from build123d import *

# Parameters (mm, degrees)
BOSS_EXTRUDE1_START = -1.5748
BOSS_EXTRUDE1_DEPTH = 126.1872
SKETCH2_R           = 5.499987026
CUT_EXTRUDE1_DEPTH  = 63.5


with BuildPart() as part:
    # Sketch1 → Boss-Extrude1 (new body)
    with BuildSketch(Plane.XY.offset(BOSS_EXTRUDE1_START)):
        with BuildLine():
            Line((5.5372, 43.3324), (35.215013396, -3.286034747))
            ThreePointArc((35.215013396, -3.286034747), (36.732607503, -7.536738968), (36.259288034, -12.025340858))
            Line((36.259288034, -12.025340858), (35.882961927, -13.127438743))
            ThreePointArc((35.882961927, -13.127438743), (33.545277751, -16.934256169), (29.80068515, -19.370370386))
            Line((29.80068515, -19.370370386), (5.435919899, -28.405771229))
            Line((5.435919899, -28.405771229), (5.401855854, -25.709375395))
            Line((5.401855854, -25.709375395), (28.91752571, -16.988852088))
            ThreePointArc((28.91752571, -16.988852088), (31.725970161, -15.161766425), (33.479233293, -12.306653356))
            Line((33.479233293, -12.306653356), (33.8555594, -11.204555471))
            ThreePointArc((33.8555594, -11.204555471), (34.210549002, -7.838104053), (33.072353421, -4.650075887))
            Line((33.072353421, -4.650075887), (3.394540025, 41.96835886))
            Line((3.394540025, 41.96835886), (5.5372, 43.3324))
        make_face()
    extrude(amount=-BOSS_EXTRUDE1_DEPTH)

    # Sketch2 → Cut-Extrude1 (cut)
    with BuildSketch(Plane(origin=(23.570559322, 15.005279885, 0), x_dir=(0, 0, -1), z_dir=(0.843566919, 0.537024071, 0))):
        with Locations((64.6684, 15.22665607)):
            Circle(SKETCH2_R)
    extrude(amount=-CUT_EXTRUDE1_DEPTH, mode=Mode.SUBTRACT)


solid = part.part
Read the model definition and answer for the solid it produces. Units are mm, in the model's axes. A direction names the side the tool comes from. Coordinates: 2 decimals unless noted, no trailing zeros. Write each loop counter-clockwise with the first axis right and the second up, starting at its lowest first coordinate (ties: lowest second). Pieces come first, ordered by that corner, then holes. Notation, with made-up numbers: M -38.75,-27 L -4.75,-27 A22 ccw -4.75,-6 Z; hole C 25.25,19 d11. An arc over 180 degrees is marked long. Use a Markdown table: item, result.
Q1. The part is cut by section C-C, the plane y = -22. Write down the section's boundary in (x, z), then the cut area to 3 significant figures.
Answer block:
| item | result |
|---|---|
| outline | M 15.4,-127.76 L 22.71,-127.76 L 22.71,-1.57 L 15.4,-1.57 Z |
| area | 922 mm2 |
Q2. Each of these flat-tipped pins is pushed along its axis until it touches: pin 1 Ø8 at (y, z) = (-8.5, -77.5) entering from -X; pin 2 Ø10 at (x, z) = (15, -48) entering from -Y; pin 3 Ø1 at (x, z) = (27.5, -64.5) entering from -Y. Where does it stop, or does it pass through?
Answer block:
| item | result |
|---|---|
| pin 1 | stops at x = 32.98 |
| pin 2 | stops at y = -26.71 |
| pin 3 | stops at y = -20.41 |
Q3. The part is cut by section B-B, the plane z = -73. Write down the section's boundary in (x, y), then the cut area to 3 significant figures.
Answer block:
| item | result |
|---|---|
| outline | M 3.39,41.97 L 33.07,-4.65 A7.62 cw 33.86,-11.2 L 33.48,-12.31 A7.62 cw 28.92,-16.99 L 5.4,-25.71 L 5.44,-28.41 L 29.8,-19.37 A10.16 ccw 35.88,-13.13 L 36.26,-12.03 A10.16 ccw 35.22,-3.29 L 5.54,43.33 Z |
| area | 248 mm2 |
Q4. Straight lines are drawn through the part: L1, parallel to Y at x = 27.5, z = -121.5; L2, parallel to Y at x = 21, z = -42.5; L3, parallel to X at y = -4.5, z = -35.5. For each, find the intervals that lie inside material, in ascending order. Write a range as [from, to].
Answer block:
| item | result |
|---|---|
| L1 | y = [-20.22, -17.51], [4.1, 8.83] |
| L2 | y = [-22.63, -19.92], [14.31, 19.04] |
| L3 | x = [32.98, 35.88] |
Q5. Determine the mould class of faces 1 (the face through (28, 5, -1.575)), 2 (the face through (36.725, -7.473, -63.785)), 3 (the face through (13.4, 28.6, -69.9)) for opening direction Z: released by +Z, released by -Z, zero draft, split by the parting line, or undercut.
Answer block:
| item | result |
|---|---|
| face 1 | released by +Z |
| face 2 | zero draft |
| face 3 | undercut |
Q6. Which of the six approach directions +Z, -Z, +X, -X, +Y, -Y give full straight-line access (tool end or side, diameter ignored) to faces 4 (the face through (17, -21.41, -63.79)), 5 (the face through (28, 5, -127.762))?
Answer block:
| item | result |
|---|---|
| face 4 | +Z, -Z, -X |
| face 5 | -Z, +X, -X, +Y, -Y |
Q7. The part is cut by section D-D, the plane y = 0. Write down the section's boundary in (x, z).
Answer block:
| item | result |
|---|---|
| outline | M 30.11,-127.76 L 33.12,-127.76 L 33.12,-1.57 L 30.11,-1.57 Z |
Q8. The part is cut by section A-A, the plane x = 22.5. Write down the section's boundary in (y, z), then the cut area to 3 significant figures.
Answer block:
| item | result |
|---|---|
| outline | M -22.08,-127.76 L -19.37,-127.76 L -19.37,-1.57 L -22.08,-1.57 Z; M 11.96,-127.76 L 16.69,-127.76 L 16.69,-1.57 L 11.96,-1.57 Z |
| area | 939 mm2 |
